from build123d import *

# Parameters (mm, degrees)
SKETCH_1_R                = 2.5
EXTRUDE_1_DEPTH           = 8.5
CUT_EXTRUDE_1_DEPTH       = 17
CUT_EXTRUDE_2_DEPTH       = 3
FILLET_1_R                = 2.5
FILLET_1_OF_MIRROR_1_R    = 2.5
CUT_EXTRUDE_3_REACH       = 19.621
SKETCH_4_R                = 2.1
HOLE_WIZARD_M2_5_1_REACH  = 22.839
HOLE_WIZARD_M2_5_1_BORE_R = 1.025
CUT_EXTRUDE_4_REACH       = 22.839
CUT_EXTRUDE_4_END_RADIUS  = 2.1
SKETCH_9_R                = 1.425
CUT_EXTRUDE_5_DEPTH       = 5.1
CUT_EXTRUDE_6_DEPTH       = 3.6


with BuildPart() as part:
    # 草图1 → 凸台-拉伸1 (new, symmetric)
    with BuildSketch(Plane.XY):
        with BuildLine():
            Line((0, 0), (0, 2.5))
            ThreePointArc((0, 2.5), (4, 6.5), (8, 2.5))
            Line((8, 2.5), (8, 0))
            Line((8, 0), (14, 0))
            Line((14, 0), (14, -6))
            Line((14, -6), (0, -6))
            Line((0, -6), (0, 0))
        make_face()
        with Locations((4, 2.5)):
            Circle(SKETCH_1_R, mode=Mode.SUBTRACT)
    extrude(amount=EXTRUDE_1_DEPTH, both=True)

    # 草图2 → 切除-拉伸1 (cut)
    with BuildSketch(Plane(origin=(0, 0, 0), x_dir=(1, 0, 0), z_dir=(0, 1, 0))):
        Polygon((12, 8.5), (14, 1.25), (14, 8.5), align=None)
        Polygon((14, -8.5), (14, -1.25), (12, -8.5), align=None)
    extrude(amount=-CUT_EXTRUDE_1_DEPTH, mode=Mode.SUBTRACT)

    # 草图3 → 切除-拉伸2 (cut)
    with BuildSketch(Plane.XY.offset(8.5)):
        Polygon((12, -1.5), (8.003412896, -1.5), (8.003412896, -6), (8.003412896, -6.782168113), (14.44734693, -6.782168113), (14.44734693, -1.5), align=None)
    cut_extrude_2 = extrude(amount=-CUT_EXTRUDE_2_DEPTH, mode=Mode.SUBTRACT)

    # 圆角1
    fillet_1_edges = [part.edges().sort_by_distance(p)[0] for p in [
        (8.003412896, -1.5, 7),
    ]]
    fillet(fillet_1_edges, radius=FILLET_1_R)

    # 镜向1: 切除-拉伸2 across plane
    add(cut_extrude_2.mirror(Plane.XY), mode=Mode.SUBTRACT)

    # 圆角1 of 镜向1
    fillet_1_of_mirror_1_edges = [part.edges().sort_by_distance(p)[0] for p in [
        (8.003412896, -1.5, -7),
    ]]
    fillet(fillet_1_of_mirror_1_edges, radius=FILLET_1_OF_MIRROR_1_R)

    # 草图4 → 切除-拉伸3 (cut, up to next)
    with BuildSketch(Plane(origin=(0, 0, 0), x_dir=(1, 0, 0), z_dir=(0, 1, 0)), mode=Mode.PRIVATE) as cut_extrude_3_sk1:
        with Locations(Location((11.05, 0, 0), (0, 0, 270))):
            Circle(SKETCH_4_R)
    cut_extrude_3_tool1 = extrude(cut_extrude_3_sk1.sketch, amount=-CUT_EXTRUDE_3_REACH, mode=Mode.PRIVATE) & part.part
    add(cut_extrude_3_tool1.solids().sort_by_distance((11.05, 0, 0))[0], mode=Mode.SUBTRACT)

    # M2.5 螺纹孔1 bore → M2.5 螺纹孔1 (cut, up to next)
    with BuildSketch(Plane.XY.offset(5.5), mode=Mode.PRIVATE) as hole_wizard_m2_5_1_sk1:
        with Locations((11.05, -4)):
            Circle(HOLE_WIZARD_M2_5_1_BORE_R)
    hole_wizard_m2_5_1_tool1 = extrude(hole_wizard_m2_5_1_sk1.sketch, amount=-HOLE_WIZARD_M2_5_1_REACH, mode=Mode.PRIVATE) & part.part
    add(hole_wizard_m2_5_1_tool1.solids().sort_by_distance((11.05, -4, 5.5))[0], mode=Mode.SUBTRACT)

    # 切除-拉伸4: up to this cylinder (the profile starts outside it)
    cut_extrude_4_end = Plane(origin=(11.05, -4, 0), z_dir=(0, 1, 0)) * Cylinder(CUT_EXTRUDE_4_END_RADIUS, 50.878, mode=Mode.PRIVATE)
    # 草图9 → 切除-拉伸4 (cut, up to the surface)
    with BuildSketch(Plane(origin=(0, 0, -5.5), x_dir=(-1, 0, 0), z_dir=(0, 0, -1)), mode=Mode.PRIVATE) as cut_extrude_4_sk1:
        with Locations((-11.05, -4)):
            Circle(SKETCH_9_R)
    cut_extrude_4_tool1 = extrude(cut_extrude_4_sk1.sketch, amount=-CUT_EXTRUDE_4_REACH, mode=Mode.PRIVATE) - cut_extrude_4_end
    add(cut_extrude_4_tool1.solids().sort_by_distance((11.05, -4, -5.5))[0], mode=Mode.SUBTRACT)

    # 草图10 → 切除-拉伸5 (cut)
    with BuildSketch(Plane.XY):
        with BuildLine():
            Line((0, 2.5), (1.5, 2.5))
            ThreePointArc((1.5, 2.5), (5.767766953, 4.267766953), (4, 0))
            Line((4, 0), (8, 0))
            Line((8, 0), (8, 2.5))
            ThreePointArc((8, 2.5), (4, 6.5), (0, 2.5))
        make_face()
    extrude(amount=CUT_EXTRUDE_5_DEPTH, mode=Mode.SUBTRACT)

    # 草图10<2> → 切除-拉伸6 (cut)
    with BuildSketch(Plane.XY):
        with BuildLine():
            Line((0, 2.5), (1.5, 2.5))
            ThreePointArc((1.5, 2.5), (5.767766953, 4.267766953), (4, 0))
            Line((4, 0), (8, 0))
            Line((8, 0), (8, 2.5))
            ThreePointArc((8, 2.5), (4, 6.5), (0, 2.5))
        make_face()
    extrude(amount=-CUT_EXTRUDE_6_DEPTH, mode=Mode.SUBTRACT)


solid = part.part
Work out the finished part from the listing and answer in its coordinate system (mm). A direction names the side the tool comes from. Give positions to 0.01 mm unless a question says otherwise; leave off trailing zeros. Write each loop counter-clockwise with the first axis right and the second up, starting at its lowest first coordinate (ties: lowest second). Pieces come first, ordered by that corner, then holes. Notation, with made-up numbers: (27.25, 15.5) - (86.25, 15.5) arc R21 ccw to (86.25, 40.5) - close; hole circle Ø2 at (59.25, -33.5). An arc over 180 degrees is marked (long way). One line per item, written item: value. Start each with the question number.
1. Given pin 1 (1.3 mm diameter, centred on x = 11, y = -4.5, fed in from -Z); pin 2 (2.5 mm diameter, centred on x = 11.05, y = -4, fed in from -Z); pin 3 (1.2 mm diameter, centred on y = 1.5, z = -6.5, fed in from +X), each flat-ended and moving along its own axis, determine where each tip first touches the part or whether it passes through.
2. For a pull along Y with two mould halves and no side action, classify faces 1 (the cylindrical face through (12, -4.39, 3.69)), 2 (the flat face through (6, 5, -3.6)), 3 (the cylindrical face through (3.9, 6.5, 6.8)) as +Y half, -Y half, draft (parallel to the pull), parting line (faces both ways), or undercut.
3. Consider probe 1 along Z at (x, y) = (1.5, 5); probe 2 along Y at (x, z) = (11.05, -4.15) (3 decimals); probe 3 along Y at (x, z) = (4, -3.75). Determine where each line is inside the solid, lowest interval first.
4. Find section A-A (x = 11.05). Write down the section's boundary in (y, z) (3 decimals).
5. Find section C-C (y = 1.5). Write down the section's boundary in (x, z), then the cut area to 3 significant figures.
6. Find section B-B (z = 0). Write down the section's boundary in (x, y), then the cut area to 3 significant figures.
7. For faces 4 (the flat face through (8, 1, -6)), 5 (the flat face through (8.003, -5, 7)), 6 (the flat face through (9, -4, -5.5)), determine the directions among +Z, -Z, +X, -X, +Y, -Y from which every point of the face is accessible in a straight line to the end or side of a thin tool.
8. Find section D-D (x = 6). Write down the section's boundary in (y, z).
Geometry results:
1. pin 1: z = 2.01
1. pin 2: z = 1.69
1. pin 3: x = 8
2. face 1: undercut
2. face 2: draft
2. face 3: +Y half
3. probe 1: -8.5 to -3.6, 5.1 to 8.5
3. probe 2: -6 to -5.425, -2.575 to 0
3. probe 3: -6 to 0, 5 to 6.5
4. outline: (-6, -5.5) - (-5.425, -5.5) - (-5.425, -2.1) - (-6, -2.1) - close; (-6, 2.1) - (-5.025, 2.1) - (-5.025, 5.5) - (-6, 5.5) - close; (-2.975, 2.1) - (0, 2.1) - (0, 8.5) - (-1.5, 8.5) - (-1.5, 5.5) - (-2.975, 5.5) - close; (-2.575, -5.5) - (-1.5, -5.5) - (-1.5, -8.5) - (0, -8.5) - (0, -2.1) - (-2.575, -2.1) - close
5. outline: (0, -8.5) - (1.71, -8.5) - (1.71, 8.5) - (0, 8.5) - close; (6.29, -8.5) - (8, -8.5) - (8, -3.6) - (6.29, -3.6) - close; (6.29, 5.1) - (8, 5.1) - (8, 8.5) - (6.29, 8.5) - close
5. area: 43.2 mm2
6. outline: (0, -6) - (8.95, -6) - (8.95, 0) - (4, 0) arc R2.5 cw to (1.5, 2.5) - (0, 2.5) - close; (13.15, -6) - (14, -6) - (14, 0) - (13.15, 0) - close
6. area: 63.9 mm2
7. face 4: +Z, -Z, +X, +Y
7. face 5: +Z, +X, -Y
7. face 6: -Z, +X, -Y
8. outline: (-6, -8.5) - (1, -8.5) - (1, -3.6) - (0, -3.6) - (0, 5.1) - (1, 5.1) - (1, 8.5) - (-6, 8.5) - close; (4, -8.5) - (5.96, -8.5) - (5.96, -3.6) - (4, -3.6) - close; (4, 5.1) - (5.96, 5.1) - (5.96, 8.5) - (4, 8.5) - close
